from build123d import *

# Parameters (mm, degrees)
SKETCH1_W           = 19.7
SKETCH1_H           = 9.7
BOSS_EXTRUDE1_DEPTH = 30
SKETCH2_W           = 39.7
SKETCH2_H           = 9.7
BOSS_EXTRUDE2_DEPTH = 10
SKETCH3_W           = 19.7
SKETCH3_H           = 4
CUT_EXTRUDE1_DEPTH  = 10
FILLET1_R           = 3
FILLET2_R           = 3


with BuildPart() as part:
    # Sketch1 → Boss-Extrude1 (new body)
    with BuildSketch(Plane.XY):
        Rectangle(SKETCH1_W, SKETCH1_H)
    extrude(amount=BOSS_EXTRUDE1_DEPTH)

    # Sketch2 → Boss-Extrude2 (add)
    with BuildSketch(Plane(origin=(0, 0, 0), x_dir=(-1, 0, 0), z_dir=(0, 0, -1))):
        Rectangle(SKETCH2_W, SKETCH2_H)
    extrude(amount=BOSS_EXTRUDE2_DEPTH)

    # Sketch3 → Cut-Extrude1 (cut)
    with BuildSketch(Plane(origin=(0, 4.85, 0), x_dir=(1, 0, 0), z_dir=(0, 1, 0))):
        with Locations((0, 5)):
            Rectangle(SKETCH3_W, SKETCH3_H)
    extrude(amount=-CUT_EXTRUDE1_DEPTH, mode=Mode.SUBTRACT)

    # Fillet1
    fillet1_edges = [part.edges().sort_by_distance(p)[0] for p in [
        (-9.85, -4.85, -5),
        (0, -4.85, -7),
        (9.85, -4.85, -5),
        (-9.85, 4.85, -5),
        (9.85, 4.85, -5),
        (0, 4.85, -7),
    ]]
    fillet(fillet1_edges, radius=FILLET1_R - 0.0001)  # a hair under: the kernel refuses the full size

    # Fillet2
    fillet2_edges = [part.edges().sort_by_distance(p)[0] for p in [
        (9.85, 0, 30),
        (0, 4.85, 30),
        (-9.85, 0, 30),
        (0, -4.85, 30),
    ]]
    fillet(fillet2_edges, radius=FILLET2_R)


solid = part.part
Geometry: final body of the model. Coordinates: model frame, mm. A direction names the side the tool comes from. Give positions to 0.01 mm unless a question says otherwise; leave off trailing zeros. Loops run counter-clockwise (first coordinate to the right, second up) from the corner with the lowest first, then second, coordinate; pieces in that order, holes last. Notation, with made-up numbers: M -36,-17.75 L -14,-17.75 A22 cw -14,14.25 Z; hole C 43.25,80.5 d1. An arc over 180 degrees is marked long. Put each result on its own line as item: value. Start each with the question number.
1) Contact query for flat-ended pins moving along their axis: pin 1 (2 mm diameter, centred on y = -0.5, z = 21, fed in from -X); pin 2 (1.5 mm diameter, centred on x = 8.5, y = -2.5, fed in from +Z); pin 3 (5 mm diameter, centred on y = 2, z = 18.5, fed in from +X). Output: stop coordinate, or through.
2) Pull-direction query (X, two-part tool) for faces 1 (the flat face through (0, 0, -10)), 2 (the cylindrical face through (9.33, 0.07, 28.69)), 3 (the flat face through (0, 0, -7)); classes: pulls with the +X half, pulls with the -X half, needs draft (parallel to the pull), parting line crosses it, or undercut.
3) Cut plane B-B (y = -1.25). Output: boundary loops of the cut face in (x, z), then the cut area to 3 significant figures.
4) Ray query, line 1 along X through (y, z) = (0.25, -5); line 2 along Z through (x, y) = (-4, 1.5); line 3 along Z through (x, y) = (8.5, 0). Return the intervals inside material, ascending.
5) Cut plane D-D (z = 12). Output: boundary loops of the cut face in (x, y), then the cut area to 3 significant figures.
6) Access query for faces 4 (the flat face through (-9.85, 0, 13)), 5 (the flat face through (9.85, 0, 13)), 6 (the cylindrical face through (-11.16, -4.33, -5.77)). Directions: +Z, -Z, +X, -X, +Y, -Y. A direction counts if a zero-diameter tool reaches every point of the face in a straight line with its end or side. Return the directions, or none.
Verdict:
1. pin 1: x = -9.85
1. pin 2: z = 29.86
1. pin 3: x = 9.85
2. face 1: needs draft
2. face 2: pulls with the +X half
2. face 3: undercut
3. outline: M -19.85,-10 L 19.85,-10 L 19.85,0 L 9.85,0 L 9.85,27 A3 ccw 6.85,30 L -6.85,30 A3 ccw -9.85,27 L -9.85,0 L -19.85,0 Z; hole M -9.85,-7 L 9.85,-7 L 9.85,-3 L -9.85,-3 Z
3. area: 905 mm2
4. line 1: -19.85 to -9.85, 9.85 to 19.85
4. line 2: -10 to -7, -3 to 30
4. line 3: -10 to -7, -3 to 29.51
5. outline: M -9.85,-4.85 L 9.85,-4.85 L 9.85,4.85 L -9.85,4.85 Z
5. area: 191 mm2
6. face 4: +Z, -X, +Y, -Y
6. face 5: +Z, +X, +Y, -Y
6. face 6: -Y
